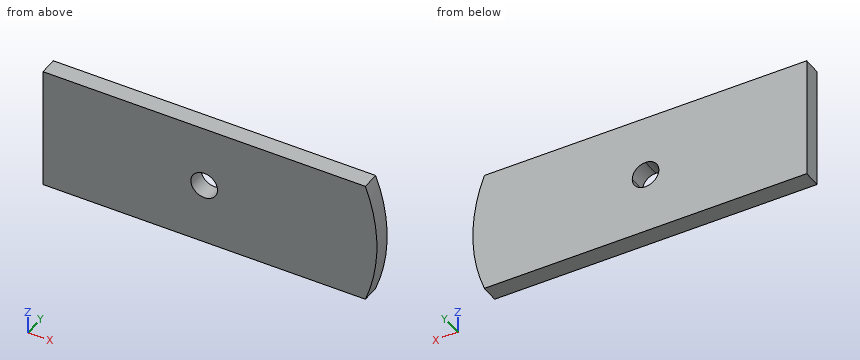
from build123d import *

# Parameters (mm, degrees)
AUFSATZ_LINEAR_AUSTRAGEN1_DEPTH = 20


with BuildPart() as part:
    # Skizze1 → Aufsatz-Linear austragen1 (new body)
    with BuildSketch(Plane(origin=(0, 0, 0), x_dir=(1, 0, 0), z_dir=(0, 1, 0))):
        with BuildLine():
            Line((182.002747232, 70), (-182.002747232, 70))
            Line((-182.002747232, 70), (-182.002747232, -70))
            Line((-182.002747232, -70), (182.002747232, -70))
            ThreePointArc((182.002747232, -70), (195, 0), (182.002747232, 70))
        make_face()
        with BuildLine():
            ThreePointArc((15.05, 0), (-10.641957057, 10.641957057), (0, -15.05))
            ThreePointArc((0, -15.05), (10.641957057, -10.641957057), (15.05, 0))
        make_face(mode=Mode.SUBTRACT)
    extrude(amount=AUFSATZ_LINEAR_AUSTRAGEN1_DEPTH)


solid = part.part
Geometry check sheet. Reference: the model listing, model coordinates, mm. Round coordinates to 2 decimals unless told otherwise and drop trailing zeros. Order: outer loops, then holes, each group sorted by start corner. A loop starts at its lowest first (then second) coordinate and runs counter-clockwise, first axis right, second up. Notation, with made-up numbers: (0.5, -2) - (6.5, -2) arc R35 ccw to (6.5, 33) - close; hole circle Ø9 at (49, 9). An arc over 180 degrees is marked (long way). One line per question, with ' | ' between items. Start each with the question number.
(1) Sectioned sample at C-C on z = -7.5. Record the cut outline in (x, y), and give its area (3 significant figures).
(2) Sectioned sample at A-A on y = 13.75. Record the cut outline in (x, z).
(3) Sectioned sample at B-B on x = -6. Record the cut outline in (y, z).
(4) Depth check by flat-ended pin: pin 1 Ø2 at (y, z) = (12.5, -20.5) entering from +X. Enter the tip coordinate at first touch or a pass-through.
(5) Thickness scan on L1, parallel to Z at x = 0, y = 8; L2, parallel to X at y = 19.25, z = 30.5; L3, parallel to X at y = 15, z = 29.5. Record the ranges inside material, lowest first. Write a range as [from, to].
Conclusion:
1) outline: (-182, 0) - (-13.05, 0) - (-13.05, 20) - (-182, 20) - close; (13.05, 0) - (194.86, 0) - (194.86, 20) - (13.05, 20) - close | area: 7,020 mm2
2) outline: (-182, -70) - (182, -70) arc R195 ccw to (182, 70) - (-182, 70) - close; hole circle Ø30.1 at (0, 0)
3) outline: (0, -70) - (20, -70) - (20, -13.8) - (0, -13.8) - close; (0, 13.8) - (20, 13.8) - (20, 70) - (0, 70) - close
4) pin 1: stops at x = 194.02
5) L1: z = [-70, -15.05], [15.05, 70] | L2: x = [-182, 192.6] | L3: x = [-182, 192.76]
